Here's the drawing with two shaded views (mm, measured from the low corner). I have some questions. A direction names the side the tool comes from. Give positions to 0.01 mm unless a question says otherwise; leave off trailing zeros. Loops run counter-clockwise (first coordinate to the right, second up) from the corner with the lowest first, then second, coordinate; pieces in that order, holes last. Notation, with made-up numbers: (-24.5, -3) -> (9.5, -3) arc R21 cw to (9.5, 27) -> close; hole circle Ø8 at (-23, -9). An arc over 180 degrees is marked (long way). Write each question's results on one line, items separated by ' | '. Start each with the question number.
Q1. If we section it at A-A, the plane z = 57: List the corners of the cut face in (x, y) for me.
Q2. If I drill on line 1 along X through (y, z) = (7, 62.5), over which ranges is the centre line in solid material (lowest first)?
Q3. Will these pins go through, and if not, where does the flat tip stop? P1, Ø3, axis at y = 26, z = 41, coming from the +X side; P2, Ø8, axis at x = 43.5, z = 28, coming from the +Y side.
Q4. Which directions (+Z, -Z, +X, -X, +Y, -Y) give clear straight access to the entire face, cutting with the end or side of a thin tool? Please do the marked faces 1 and 2.
Q5. If we section it at B-B, the plane x = 47.5: List the corners of the cut face in (y, z) for me.
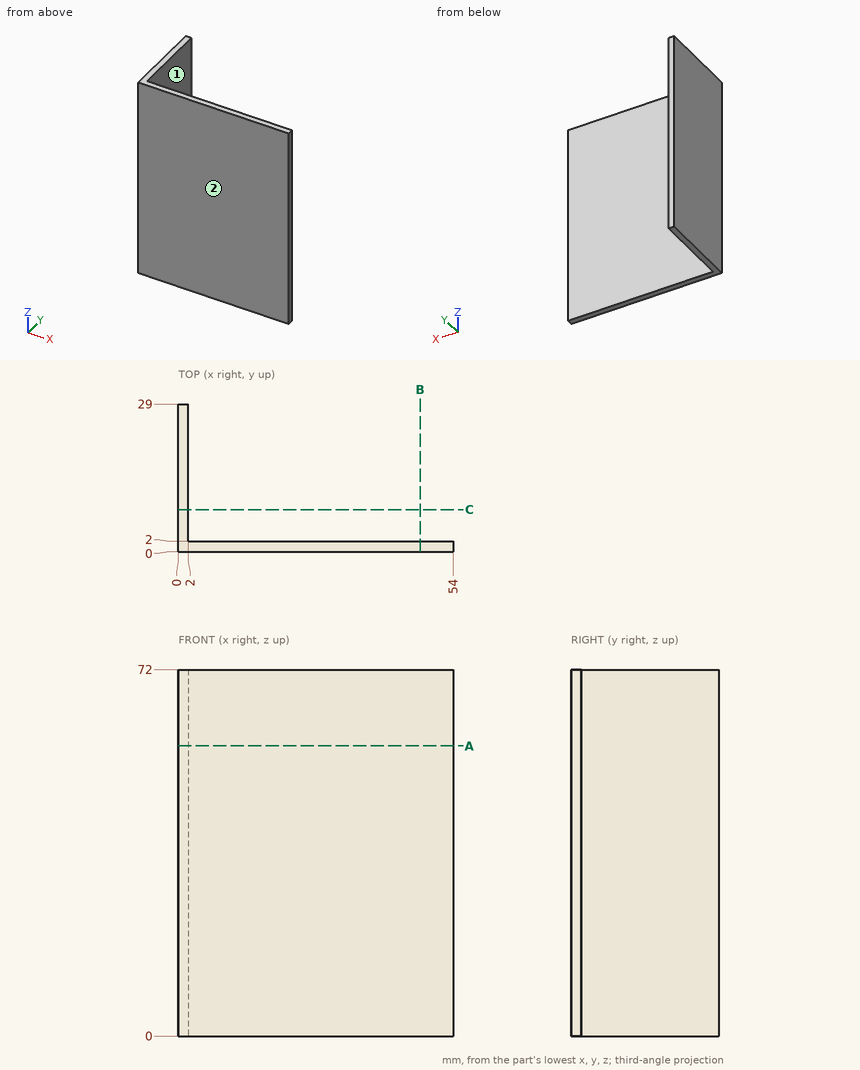
Final values:
1) outline: (0, 0) -> (54, 0) -> (54, 2) -> (2, 2) -> (2, 29) -> (0, 29) -> close
2) line 1: x = 0 to 2
3) P1: stops at x = 2 | P2: stops at y = 2
4) face 1: +Z, -Z, +X, +Y | face 2: +Z, -Z, +X, -X, -Y
5) outline: (0, 0) -> (2, 0) -> (2, 72) -> (0, 72) -> close
